Autodesk Inventor part; units mm, degrees
ref_plane "YZ Plane" through (0, 0, 0) normal (1, 0, 0) x (0, 1, 0)
ref_plane "XZ Plane" through (0, 0, 0) normal (0, 1, 0) x (-1, 0, 0)
ref_plane "XY Plane" through (0, 0, 0) normal (0, 0, 1) x (1, 0, 0)
sketch "Skizze1" plane through (0, 0, 0) normal (0, 0, 1) x (1, 0, 0)
  line L0 (-60, -26.5) -> (60, -26.5)
  line L1 (60, -26.5) -> (60, 26.5)
  line L2 (60, 26.5) -> (-60, 26.5)
  line L3 (-60, 26.5) -> (-60, -26.5)
  line L4 (-60, -26.5) -> (60, 26.5) construction
  line L5 (60, -26.5) -> (-60, 26.5) construction
  point P0 (0, 0)
  dimension "d0" = 53
  dimension "d1" = 120
extrude "Extrusion1" add sketch "Skizze1" along normal blind 4
sketch "Skizze2" plane through (0, 0, 0) normal (0, 0, -1) x (-1, 0, 0)
  line L0 (-60, -23.5) -> (-60, -26.5) construction
  line L1 (-54, -4) -> (-56.5, -4)
  line L2 (-56.5, -4) -> (-56.5, 1)
  line L3 (-56.5, 1) -> (-54, 1)
  line L4 (-54, 1) -> (-54, -4)
  line L5 (-54, -4) -> (-56.5, 1) construction
  line L6 (-56.5, -4) -> (-54, 1) construction
  line L7 (54, -1) -> (56.5, -1)
  line L8 (56.5, -1) -> (56.5, 4)
  line L9 (56.5, 4) -> (54, 4)
  line L10 (54, 4) -> (54, -1)
  line L11 (54, -1) -> (56.5, 4) construction
  line L12 (56.5, -1) -> (54, 4) construction
  line L13 (60, -26.5) -> (-60, -26.5)
  point P0 (0, 0)
  point P1 (-55.25, -1.5)
  point P2 (-55.25, -1.5)
  dimension "d5" = 2.5
  dimension "d6" = 5
  dimension "d68" = 25
extrude "Extrusion2" add sketch "Skizze2" along normal blind 15 contours L1 L2 L3 L4
sketch "Skizze6" plane through (56.5, -4, 0) normal (1, 0, 0) x (0, 0, -1)
  line L0 (15, 5) -> (15, 0)
  line L1 (15, 2.5) -> (0, 2.5)
  line L2 (0, -22.5) -> (0, 30.5)
  line L3 (10.5, 0) -> (15, 0)
  line L4 (15, 0) -> (15, 5)
  line L5 (15, 5) -> (10.5, 5)
  line L6 (10.5, 5) -> (10.5, 0)
  line L7 (10.5, 0) -> (15, 5) construction
  line L8 (15, 0) -> (10.5, 5) construction
  point P0 (0, 4)
  point P1 (12.75, 2.5)
  point P2 (15, 0)
  dimension "d19" = 4.5
  dimension "d20" = 5
extrude "Extrusion5" add sketch "Skizze6" along normal blind 3.5
mirror "Spiegeln2" about plane through (0, 0, 0) normal (1, 0, 0) of "Extrusion2", "Extrusion5"
sketch "Skizze7" plane through (0, 0, 4) normal (0, 0, 1) x (1, 0, 0)
  line L0 (-26.5, -12.5) -> (46.5, -12.5)
  line L1 (46.5, -12.5) -> (46.5, 12.5)
  line L2 (46.5, 12.5) -> (-26.5, 12.5)
  line L3 (-26.5, 12.5) -> (-26.5, -12.5)
  line L4 (-26.5, -12.5) -> (46.5, 12.5) construction
  line L5 (46.5, -12.5) -> (-26.5, 12.5) construction
  point P0 (0, 0)
  point P1 (10, 0)
  dimension "d23" = 10
  dimension "d24" = 73
  dimension "d25" = 25
extrude "Extrusion6" cut sketch "Skizze7" against normal through all
sketch "Skizze8" plane through (0, 0, 4) normal (0, 0, 1) x (1, 0, 0)
  line L0 (-60, 26.5) -> (-60, -26.5)
  line L1 (-60, 0) -> (60, 0)
  line L2 (60, -26.5) -> (60, 26.5)
  line L3 (-56, 10) -> (-26.5, 10) construction
  line L4 (-26.5, -12.5) -> (-26.5, 12.5) construction
  circle A0 centre (-45, 10) radius 1.25
  line L5 (-40, 10) -> (-40, 12.8313) construction
  circle A1 centre (-35, 10) radius 1.25
  line L6 (-40, 10) -> (-40, 0) construction
  line L7 (-43.5, 1.5) -> (-36.5, 1.5) construction
  line L8 (-43.5, 0) -> (-36.5, 0)
  line L9 (-36.5, 3) -> (-43.5, 3)
  arc A2 (-43.5, 3) -> (-43.5, 0) centre (-43.5, 1.5) ccw
  arc A3 (-36.5, 0) -> (-36.5, 3) centre (-36.5, 1.5) ccw
  point P0 (0, 0)
  point P1 (-26.5, 0)
  point P2 (-40, 1.5)
  dimension "d28" = 10
  dimension "d29" = 2.5
  dimension "d30" = 10
  dimension "d31" = 7
  dimension "d55" = 13.5
  dimension "d69" = 3
extrude "Extrusion7" cut sketch "Skizze8" against normal blind 10
sketch "Skizze9" plane through (0, 0, 4) normal (0, 0, 1) x (1, 0, 0)
  circle A0 centre (-28, 17) radius 2.25
  line L0 (-26.5, 12.5) -> (46.5, 12.5)
  line L1 (46.5, 12.5) -> (-26.5, 12.5)
  line L2 (10, 12.5) -> (10, -12.5)
  line L3 (-25.5, 0) -> (45.5, 0)
  circle A1 centre (48, 17) radius 2.25
  circle A2 centre (-28.3, -15) radius 2.25
  line L4 (46.5, -12.5) -> (-26.5, -12.5)
  line L5 (-26.5, -12.5) -> (-26.5, 12.5)
  circle A3 centre (48.3, -15) radius 2.25
  point P0 (0, 0)
  dimension "d35" = 4.5
  dimension "d37" = 4.5
  dimension "d40" = 2.5
  dimension "d41" = 1.8
  dimension "d42" = 4.5
  dimension "d53" = 1.5
extrude "Extrusion8" cut sketch "Skizze9" against normal blind 10 contours A0 | A1 | A2 | A3
fillet "Rundung1" radius 2 4 edges at (-60, 26.5, 2) (60, 26.5, 2) (-60, -26.5, 2) (60, -26.5, 2)
fillet "Rundung4" radius 0.8 4 edges at (56.5, -1.5, -10.5) (54, -1.5, -15) (-54, -1.5, -15) (-56.5, -1.5, -10.5)
fillet "Rundung5" radius 2 4 edges at (55.25, 1, 0) (55.25, -4, 0) (-55.25, 1, 0) (-55.25, -4, 0)
chamfer "Fase4" distance 2 angle 45 2 edges at (60, -1.5, -15) (-60, -1.5, -15)
sketch "Skizze11" plane through (0, 0, 4) normal (0, 0, 1) x (1, 0, 0)
  line L0 (-36.5, 0) -> (-43.5, 0) construction
  line L1 (-40, 0) -> (-40, -26.5) construction
  line L2 (-58, -26.5) -> (58, -26.5) construction
  circle A0 centre (-43, -8) radius 1.5
  circle A1 centre (-37, -8) radius 1.5
  line L3 (-43, -8) -> (-40, -8) construction
  line L4 (-37, -8) -> (-40, -8) construction
  point P0 (0, 0)
  dimension "d70" = 3
  dimension "d71" = 3
  dimension "d72" = 3
  dimension "d73" = 8
extrude "Extrusion10" cut sketch "Skizze11" against normal blind 10
properties part number "Front"
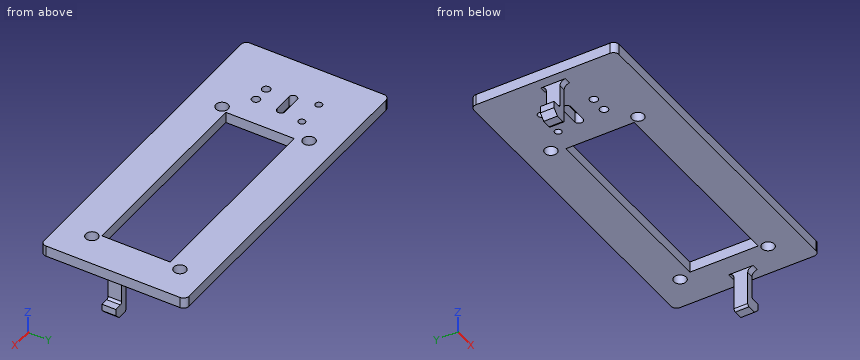
Work out the finished part from the listing and answer in its coordinate system (mm). Round coordinates to 2 decimals unless told otherwise and drop trailing zeros. Write each loop counter-clockwise with the first axis right and the second up, starting at its lowest first coordinate (ties: lowest second). Pieces come first, ordered by that corner, then holes.
1) Straight lines are drawn through the part: line 1 (Y direction, x = -28.3, z = 2.5); line 2 (X direction, y = -2.5, z = -11.75); line 3 (Y direction, x = -20, z = 1.25). For each, find the intervals that lie inside material, in ascending order.
2) Given pin 1 Ø5 at (x, y) = (48.3, -15) entering from -Z; pin 2 Ø1.8 at (x, z) = (-56.5, -10.5) entering from -Y; pin 3 Ø3 at (x, z) = (-56, -5.5) entering from +Y, each flat-ended and moving along its own axis, determine where each tip first touches the part or whether it passes through.
3) A cutting plane is placed at A-A (z = -3.5). Give the vertices of the cut face in (x, y).
4) A cutting plane is placed at D-D (y = -15). Give the vertices of the cut face in (x, z), plus the area to 3 significant figures.
5) A cutting plane is placed at B-B (x = -23.5). Give the vertices of the cut face in (y, z).
6) A cutting plane is placed at C-C (y = 10). Give the vertices of the cut face in (x, z), plus the area to 3 significant figures.
Completed:
1. line 1: y = -26.5 to -17.25, -12.75 to 14.77, 19.23 to 26.5
1. line 2: x = -60 to -54, 54 to 60
1. line 3: y = -26.5 to -12.5, 12.5 to 26.5
2. pin 1: stops at z = 0
2. pin 2: stops at y = -4
2. pin 3: stops at y = 1
3. outline: (-56.5, -4) - (-54, -4) - (-54, 1) - (-56.5, 1) - close; (54, -4) - (56.5, -4) - (56.5, 1) - (54, 1) - close
4. outline: (-60, 0) - (-30.55, 0) - (-30.55, 4) - (-60, 4) - close; (-26.05, 0) - (46.05, 0) - (46.05, 4) - (-26.05, 4) - close; (50.55, 0) - (60, 0) - (60, 4) - (50.55, 4) - close
4. area: 444 mm2
5. outline: (-26.5, 0) - (-12.5, 0) - (-12.5, 4) - (-26.5, 4) - close; (12.5, 0) - (26.5, 0) - (26.5, 4) - (12.5, 4) - close
6. outline: (-60, 0) - (-46.25, 0) - (-46.25, 4) - (-60, 4) - close; (-43.75, 0) - (-36.25, 0) - (-36.25, 4) - (-43.75, 4) - close; (-33.75, 0) - (-26.5, 0) - (-26.5, 4) - (-33.75, 4) - close; (46.5, 0) - (60, 0) - (60, 4) - (46.5, 4) - close
6. area: 168 mm2
